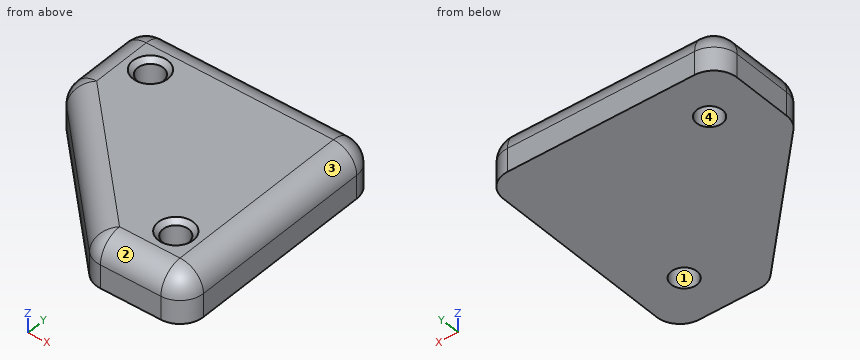
Autodesk Inventor part; units mm, degrees
ref_plane "YZ Plane" through (0, 0, 0) normal (1, 0, 0) x (0, 1, 0)
ref_plane "XZ Plane" through (0, 0, 0) normal (0, 1, 0) x (-1, 0, 0)
ref_plane "XY Plane" through (0, 0, 0) normal (0, 0, 1) x (1, 0, 0)
sketch "스케치1" plane through (0, 0, 0) normal (0, 0, 1) x (1, 0, 0)
  line L0 (5, -25) -> (25, -25)
  line L1 (25, -25) -> (25, 25)
  line L2 (25, 25) -> (-25, 25)
  line L3 (-25, 25) -> (-25, 5)
  line L4 (-10, -10) -> (25, 25) construction
  line L5 (25, -25) -> (-25, 25) construction
  line L6 (5, -25) -> (-25, 5)
  point P0 (0, 0)
  dimension "d0" = 50
  dimension "d1" = 50
  dimension "d2" = 20
  dimension "d3" = 20
extrude "돌출1" add sketch "스케치1" along normal blind 10
fillet "모깎기1" radius 5 5 edges at (25, 25, 5) (25, -25, 5) (-25, 25, 5) (-25, 5, 5) (5, -25, 5)
fillet "모깎기2" radius 5 10 edges at (23.5355, 23.5355, 10) (0, 25, 10) (-23.5355, 23.5355, 10) (-25, 13.5355, 10) (-24.6194, 5.1577, 10) (-10, -10, 10) (5.1577, -24.6194, 10) (13.5355, -25, 10) (23.5355, -23.5355, 10) (25, 0, 10)
sketch "스케치2" plane through (0, 0, 0) normal (0, 0, -1) x (-1, 0, 0)
  line L0 (25, 20) -> (25, 7.0711)
  line L1 (-20, 25) -> (20, 25)
  line L2 (-25, -20) -> (-25, 20)
  line L3 (-7.0711, -25) -> (-20, -25)
  line L4 (-15, 15) -> (15, 15) construction
  line L5 (-15, -15) -> (-15, 15) construction
  circle A0 centre (-15, -15) radius 2.75
  circle A1 centre (15, 15) radius 2.75
  point P0 (0, 0)
  point P1 (-25, 0)
  dimension "d8" = 10
  dimension "d10" = 10
  dimension "d11" = 10
  dimension "d12" = 10
  dimension "d13" = 5.5
  dimension "d14" = 5.5
extrude "돌출2" cut sketch "스케치2" against normal blind 10
chamfer "모따기1" distance 1 angle 45 2 edges at (-12.25, 15, 10) (17.75, -15, 10)
equation "\"d13\" = d14"
properties part number "모서리 결합"
The listing builds one solid part. Answer for the finished solid, in the listing's coordinates (mm). Face numbers are marked on the shaded views. Round coordinates to 2 decimals unless told otherwise and drop trailing zeros. Loops run counter-clockwise (first coordinate to the right, second up) from the corner with the lowest first, then second, coordinate; pieces in that order, holes last. Notation, with made-up numbers: M 51,87.25 L 110,87.25 A22 ccw 110,126.25 Z; hole C 67,1 d5. An arc over 180 degrees is marked long. Write each question's results on one line, items separated by ' | '. Start each with the question number.
1) Find section A-A on x = 15. Write down the section's boundary in (y, z), plus the area to 3 significant figures.
2) Straight lines are drawn through the part: probe 1 along Y at (x, z) = (15, 2); probe 2 along Y at (x, z) = (-15, 6.25); probe 3 along X at (y, z) = (12.5, 7). For each, find the intervals that lie inside material, in ascending order.
3) Find section C-C on z = 3.5. Write down the section's boundary in (x, y), plus the area to 3 significant figures.
4) Determine the mould class of the marked faces 1, 2, 3 and 4 for opening direction Y: pulls with the +Y half, pulls with the -Y half, needs draft (parallel to the pull), parting line crosses it, or undercut.
5) Find section D-D on y = 9. Write down the section's boundary in (x, z).
6) Each of these flat-tipped pins is pushed along its axis until it touches: pin 1 (2 mm diameter, centred on x = -16, z = 7.5, fed in from +Y); pin 2 (2 mm diameter, centred on x = -5.5, z = 8, fed in from -Y). Where does it stop, or does it pass through?
Final values:
1) outline: M -25,0 L -17.75,0 L -17.75,9 L -18.75,10 L -20,10 A5 ccw -25,5 Z; M -12.25,0 L 25,0 L 25,5 A5 ccw 20,10 L -11.25,10 L -12.25,9 Z | area: 433 mm²
2) probe 1: -25 to -17.75, -12.25 to 25 | probe 2: -4.78 to 12.25, 17.75 to 24.84 | probe 3: -24.58 to -16.15, -13.85 to 24.58
3) outline: M -25,7.07 A5 ccw -23.54,3.54 L 3.54,-23.54 A5 ccw 7.07,-25 L 20,-25 A5 ccw 25,-20 L 25,20 A5 ccw 20,25 L -20,25 A5 ccw -25,20 Z; hole C -15,15 d5.5; hole C 15,-15 d5.5 | area: 1,990 mm²
4) face 1: undercut | face 2: pulls with the -Y half | face 3: needs draft | face 4: undercut
5) outline: M -25,0 L 25,0 L 25,5 A5 ccw 20,10 L -20,10 A5 ccw -25,5 Z
6) pin 1: y = 24.77 | pin 2: y = -14.43
